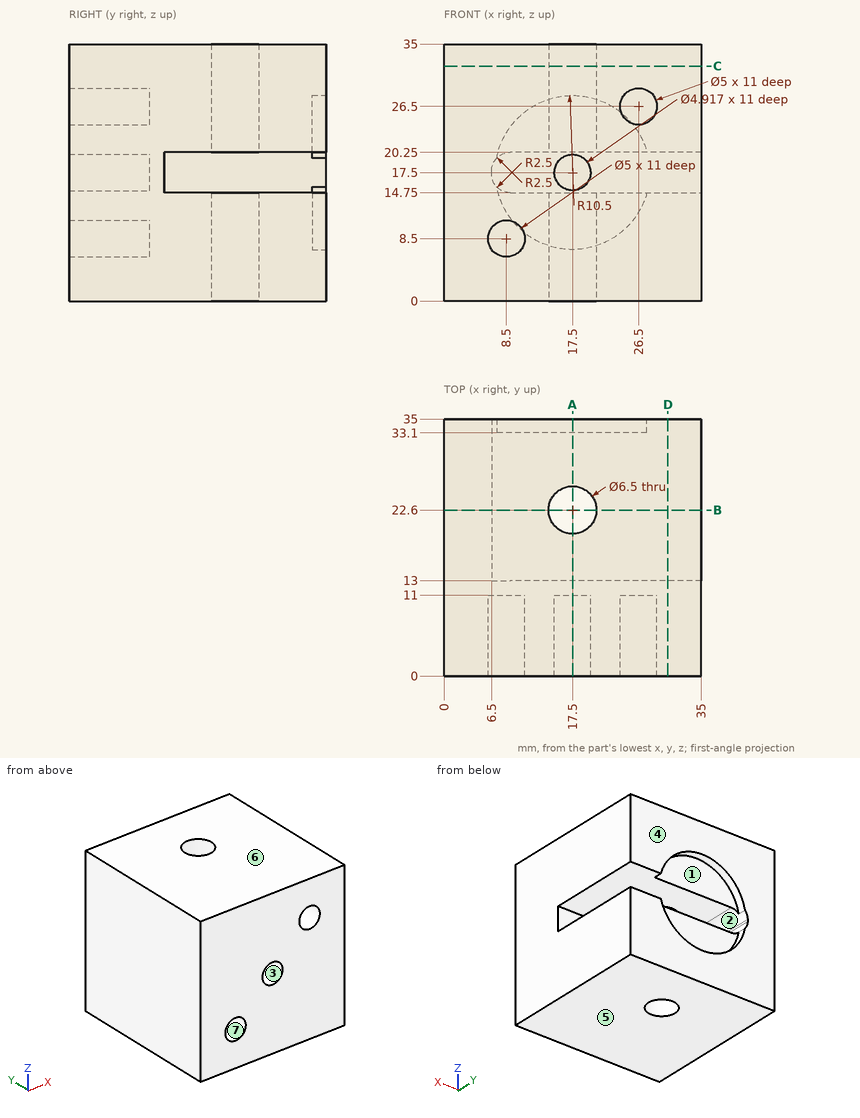
Study the drawing (mm; zero at the part's minimum x, y, z) and answer. A direction names the side the tool comes from. Give positions to 0.01 mm unless a question says otherwise; leave off trailing zeros. Write each loop counter-clockwise with the first axis right and the second up, starting at its lowest first coordinate (ties: lowest second). Pieces come first, ordered by that corner, then holes. Notation, with made-up numbers: (28, -8) - (49, -8) arc R26 cw to (49, 25) - close; hole circle Ø6 at (2, 80). An arc over 180 degrees is marked (long way). Use CSV: the item, a comma, the result in double quotes. Start each with the question number.
(1) Given P1, Ø5, axis at x = 17.5, y = 22.6, coming from the -Z side; P2, Ø0.6, axis at y = 26, z = 17.5, coming from the +X side; P3, Ø4, axis at x = 8.5, z = 8.5, coming from the -Y side; P4, Ø4.5, axis at x = 18, z = 13, coming from the +Y side, each flat-ended and moving along its own axis, determine where each tip first touches the part or whether it passes through.
(2) Find section C-C (z = 32). Give the vertices of the cut face in (x, y).
(3) Determine the mould class of the marked faces 5, 6 and 7 for opening direction Z: +Z half, -Z half, draft (parallel to the pull), parting line (faces both ways), or undercut.
(4) Find section D-D (x = 30.5). Give the vertices of the cut face in (y, z), plus the area to 3 significant figures.
(5) For the marked faces 1, 2, 3 and 4, determine the directions among +Z, -Z, +X, -X, +Y, -Y from which every point of the face is accessible in a straight line to the end or side of a thin tool.
(6) Consider line 1 along X through (y, z) = (22.6, 9.25); line 2 along Z through (x, y) = (12, 20); line 3 along X through (y, z) = (2.5, 26.5). Determine where each line is inside the solid, lowest interval first.
(7) Find section A-A (x = 17.5). Give the vertices of the cut face in (y, z).
(8) Find section B-B (y = 22.6). Give the vertices of the cut face in (x, z), plus the area to 3 significant figures.
Findings below:
1,P1,"through"
1,P2,"x = 6.5"
1,P3,"y = 11"
1,P4,"y = 33.1"
2,outline,"(0, 0) - (35, 0) - (35, 35) - (0, 35) - close; hole circle Ø6.5 at (17.5, 22.6)"
3,face 5,"-Z half"
3,face 6,"+Z half"
3,face 7,"undercut"
4,outline,"(0, 0) - (35, 0) - (35, 14.75) - (13, 14.75) - (13, 20.25) - (35, 20.25) - (35, 35) - (0, 35) - close"
4,area,"1,100 mm2"
5,face 1,"+Y"
5,face 2,"+X, +Y"
5,face 3,"-Y"
5,face 4,"+Z, -Z, +X, -X, +Y"
6,line 1,"0 to 14.25, 20.75 to 35"
6,line 2,"0 to 14.75, 20.25 to 35"
6,line 3,"0 to 24, 29 to 35"
7,outline,"(0, 0) - (19.35, 0) - (19.35, 14.75) - (13, 14.75) - (13, 20.25) - (19.35, 20.25) - (19.35, 35) - (0, 35) - (0, 19.96) - (11, 19.96) - (11, 15.04) - (0, 15.04) - close; (25.85, 0) - (35, 0) - (35, 7) - (33.1, 7) - (33.1, 14.75) - (25.85, 14.75) - close; (25.85, 20.25) - (33.1, 20.25) - (33.1, 28) - (35, 28) - (35, 35) - (25.85, 35) - close"
8,outline,"(0, 0) - (14.25, 0) - (14.25, 14.75) - (9, 14.75) arc R2.5 cw to (6.5, 17.25) - (6.5, 17.75) arc R2.5 cw to (9, 20.25) - (14.25, 20.25) - (14.25, 35) - (0, 35) - close; (20.75, 0) - (35, 0) - (35, 14.75) - (20.75, 14.75) - close; (20.75, 20.25) - (35, 20.25) - (35, 35) - (20.75, 35) - close"
8,area,"879 mm2"
